Verification items for the finished model (mm, model axes). Face numbers are marked on the shaded views. A direction names the side the tool comes from. Give positions to 0.01 mm unless a question says otherwise; leave off trailing zeros. Loops run counter-clockwise (first coordinate to the right, second up) from the corner with the lowest first, then second, coordinate; pieces in that order, holes last. Notation, with made-up numbers: (65.5, -38.5) -> (74.5, -38.5) arc R28 ccw to (74.5, -8.5) -> close; hole circle Ø8 at (-2, -11). An arc over 180 degrees is marked (long way). Answer in a Markdown table with one row per item. Add a question column.
Q1. Section check C-C on x = -6. Give the number of separate pieces and of enclosed holes in the cut face, and give its area (3 significant figures).
Q2. Release check for a two-part mould opening along Y. For the marked faces 1, 2 and 3 record: pulls with the +Y half, pulls with the -Y half, needs draft (parallel to the pull), parting line crosses it, or undercut.
Q3. Gauge pin test, flat ends, axial feed: P1, Ø8, axis at y = 9, z = 26.5, coming from the +X side; P2, Ø4, axis at x = 1, z = 6.5, coming from the +Y side; P3, Ø2, axis at x = -4.5, z = 2, coming from the -Y side. Record the tip position at first contact, or that the pin passes through.
Q4. Material ranges on probe 1 along X at (y, z) = (9, 18); probe 2 along Y at (x, z) = (-3, -30.5); probe 3 along X at (y, z) = (14, 14.5), recorded low to high.
Q5. Set-up check for the marked faces 4 and 5: record each of +Z, -Z, +X, -X, +Y, -Y from which the full face is reachable in a straight line by a thin tool's end or side.
Q6. Section check B-B on z = -2.5. Enter the section's corners in (x, y), and give its area (3 significant figures).
Q7. Section check A-A on z = -30.5. Enter the section's corners in (x, y), and give its area (3 significant figures).
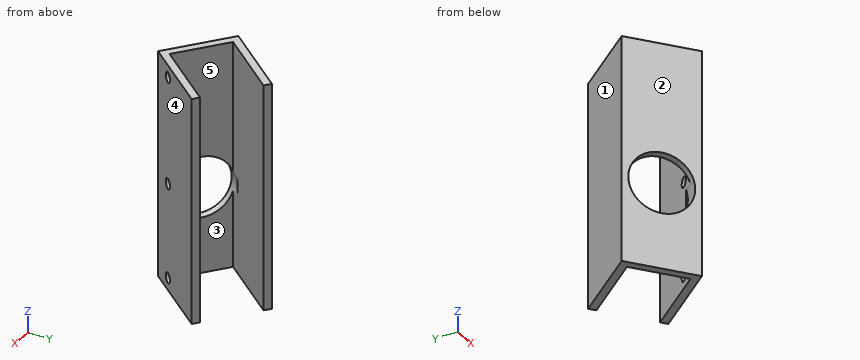
```python
from build123d import *

# Parameters (mm, degrees)
ESTRUSIONE_SOTTILE1_DEPTH      = 37
ESTRUSIONE_SOTTILE1_DEPTH_BACK = 37
SCHIZZO2_R                     = 1.7
TAGLIO_ESTRUSIONE2_DEPTH       = 23
SCHIZZO3_R                     = 10
TAGLIO_ESTRUSIONE3_DEPTH       = 6
SCHIZZO4_W                     = 19
SCHIZZO4_H                     = 35
TAGLIO_ESTRUSIONE4_DEPTH       = 9
SCHIZZO5_R                     = 1.7
TAGLIO_ESTRUSIONE5_DEPTH       = 9
TAGLIO_ESTRUSIONE6_DEPTH       = 38
TAGLIO_ESTRUSIONE6_DEPTH_BACK  = 38


with BuildPart() as part:
    # Schizzo1 → Estrusione-Sottile1 (new body, two sides)
    with BuildSketch(Plane.XY) as estrusione_sottile1_sk:
        with BuildLine():
            Line((1.3418419, 31.371953403), (-14.62198067, 12.132505153))
            Line((-14.62198067, 12.132505153), (0, 0))
            Line((0, 0), (76.626348337, 92.349351598))
            ThreePointArc((76.626348337, 92.349351598), (100.821605793, 105.569380982), (125.016863249, 92.349351598))
            Line((125.016863249, 92.349351598), (132.637123428, 81.561358928))
            Line((132.637123428, 81.561358928), (153.805626203, 63.996914357))
            Line((153.805626203, 63.996914357), (152.209243946, 62.072969532))
            Line((152.209243946, 62.072969532), (130.786083182, 79.848715119))
            Line((130.786083182, 79.848715119), (122.942210931, 90.953275114))
            ThreePointArc((122.942210931, 90.953275114), (100.774095149, 103.069337988), (78.649981188, 90.873112409))
            Line((78.649981188, 90.873112409), (0.327562568, -3.520327082))
            Line((0.327562568, -3.520327082), (-18.142307752, 11.804942585))
            Line((-18.142307752, 11.804942585), (-0.582102925, 32.96833566))
            Line((-0.582102925, 32.96833566), (1.3418419, 31.371953403))
        make_face()
    extrude(amount=ESTRUSIONE_SOTTILE1_DEPTH)
    extrude(estrusione_sottile1_sk.sketch, amount=-ESTRUSIONE_SOTTILE1_DEPTH_BACK)

    # Schizzo2 → Taglio-Estrusione2 (cut)
    with BuildSketch(Plane(origin=(1.923944825, -1.596382257, 0), x_dir=(0, 0, -1), z_dir=(0.76957793, -0.638552903, 0))):
        with Locations((-6.552412565, 114.869422042)):
            Circle(SCHIZZO2_R)
        with Locations((-6.552412565, 104.052556993)):
            Circle(SCHIZZO2_R)
        with Locations((1.452296176, 109.710473024)):
            Circle(SCHIZZO2_R)
        with Locations((9.457004918, 104.551524007)):
            Circle(SCHIZZO2_R)
        with Locations((1.553386665, 98.82845624)):
            Circle(SCHIZZO2_R)
        with Locations((9.659185895, 93.604355486)):
            Circle(SCHIZZO2_R)
    extrude(amount=-TAGLIO_ESTRUSIONE2_DEPTH, mode=Mode.SUBTRACT)

    # Schizzo3 → Taglio-Estrusione3 (cut)
    with BuildSketch(Plane(origin=(-1.596382257, -1.923944825, 0), x_dir=(0.76957793, -0.638552903, 0), z_dir=(-0.638552903, -0.76957793, 0))):
        with Locations((-9.5, -8.811563563)):
            Circle(SCHIZZO3_R)
    extrude(amount=-TAGLIO_ESTRUSIONE3_DEPTH, mode=Mode.SUBTRACT)

    # Schizzo4 → Taglio-Estrusione4 (cut)
    with BuildSketch(Plane(origin=(0, 0, 0), x_dir=(0, 0, 1), z_dir=(-0.76957793, 0.638552903, 0))):
        with Locations((-7.5, 57.5)):
            Rectangle(SCHIZZO4_W, SCHIZZO4_H)
    extrude(amount=-TAGLIO_ESTRUSIONE4_DEPTH, mode=Mode.SUBTRACT)

    # Schizzo5 → Taglio-Estrusione5 (cut)
    with BuildSketch(Plane(origin=(0, 0, 0), x_dir=(0, 0, 1), z_dir=(-0.76957793, 0.638552903, 0))):
        with Locations((33, 5.5)):
            Circle(SCHIZZO5_R)
        with Locations((-33, 5.5)):
            Circle(SCHIZZO5_R)
        with Locations((-2, 5.5)):
            Circle(SCHIZZO5_R)
    extrude(amount=-TAGLIO_ESTRUSIONE5_DEPTH, mode=Mode.SUBTRACT)

    # Schizzo6 → Taglio-Estrusione6 (cut, two sides)
    with BuildSketch(Plane.XY) as taglio_estrusione6_sk:
        Polygon((1.3418419, 31.371953403), (32.99116726, 5.111106005), (167.345945228, 57.415127601), (141.955436185, 113.188092886), (32.984624639, 110.825582067), align=None)
    extrude(amount=TAGLIO_ESTRUSIONE6_DEPTH, mode=Mode.SUBTRACT)
    extrude(taglio_estrusione6_sk.sketch, amount=-TAGLIO_ESTRUSIONE6_DEPTH_BACK, mode=Mode.SUBTRACT)


solid = part.part
```
Taken from the geometry:
| question | item | result |
|---|---|---|
| 1 | separate pieces | 3 |
| 1 | enclosed holes | 0 |
| 1 | area | 468 mm² |
| 2 | face 1 | pulls with the +Y half |
| 2 | face 2 | pulls with the -Y half |
| 2 | face 3 | undercut |
| 3 | P1 | stops at x = 14.04 |
| 3 | P2 | stops at y = 32.97 |
| 3 | P3 | stops at y = -0.34 |
| 4 | probe 1 | x = -14.76 to -10.85, 7.47 to 10.72 |
| 4 | probe 2 | y = -0.76 to 2.49, 26.14 to 30.05 |
| 4 | probe 3 | x = -16.32 to -13.07, 11.62 to 14.86 |
| 5 | face 4 | +Z, -Z, +X, -Y |
| 5 | face 5 | +Z, -Z |
| 6 | outline | (-18.14, 11.8) -> (-14.88, 9.1) -> (-13.28, 11.02) -> (-14.62, 12.13) -> (1.34, 31.37) -> (-0.58, 32.97) -> close; (-2.94, -0.81) -> (0.33, -3.52) -> (4.4, 1.39) -> (2.47, 2.98) -> (0, 0) -> (-1.34, 1.11) -> close; (4.55, 5.48) -> (6.47, 3.89) -> (17.89, 17.64) -> (15.96, 19.24) -> close |
| 6 | area | 138 mm² |
| 7 | outline | (-18.14, 11.8) -> (0.33, -3.52) -> (17.89, 17.64) -> (15.96, 19.24) -> (0, 0) -> (-14.62, 12.13) -> (1.34, 31.37) -> (-0.58, 32.97) -> close |
| 7 | area | 185 mm² |
